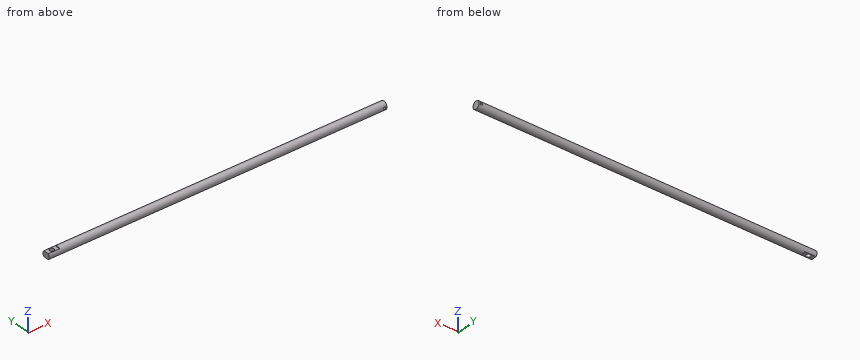
from build123d import *

# Parameters (mm, degrees)
SKETCH_1_R           = 7
EXTRUDE_1_DEPTH      = 600
SKETCH_3_OUTSIDE_W   = 136.066
SKETCH_3_OUTSIDE_H   = 136.066
SKETCH_3_OUTSIDE_W_2 = 10
SKETCH_3_OUTSIDE_H_2 = 20
CUT_EXTRUDE_1_DEPTH  = 20
SKETCH_4_R           = 4
CUT_EXTRUDE_3_DEPTH  = 20
SKETCH_5_R           = 2
CUT_EXTRUDE_4_DEPTH  = 15


with BuildPart() as part:
    # 草图1 → 凸台-拉伸1 (new body)
    with BuildSketch(Plane(origin=(0, 0, 0), x_dir=(0, 0, -1), z_dir=(1, 0, 0))):
        Circle(SKETCH_1_R)
    extrude(amount=EXTRUDE_1_DEPTH)

    # 草图3 outside → 切除-拉伸1 (cut)
    with BuildSketch(Plane.ZY):
        Rectangle(SKETCH_3_OUTSIDE_W, SKETCH_3_OUTSIDE_H)
        Rectangle(SKETCH_3_OUTSIDE_W_2, SKETCH_3_OUTSIDE_H_2, mode=Mode.SUBTRACT)
    extrude(amount=-CUT_EXTRUDE_1_DEPTH, mode=Mode.SUBTRACT)

    # 草图4 → 切除-拉伸3 (cut)
    with BuildSketch(Plane(origin=(0, 0, -5), x_dir=(-1, 0, 0), z_dir=(0, 0, -1))):
        with Locations((-10, 0)):
            Circle(SKETCH_4_R)
    extrude(amount=-CUT_EXTRUDE_3_DEPTH, mode=Mode.SUBTRACT)

    # 草图5 → 切除-拉伸4 (cut, through all)
    with BuildSketch(Plane(origin=(-583.138159927, 7, 1388.026133711), x_dir=(-1, 0, 0), z_dir=(0, 1, 0))):
        with Locations((-1179.138160513, -1388.026133214)):
            Circle(SKETCH_5_R)
    extrude(amount=-CUT_EXTRUDE_4_DEPTH, mode=Mode.SUBTRACT)


solid = part.part
CAD build for the part. Positions are in the model's coordinates, mm. Round coordinates to 2 decimals unless told otherwise and drop trailing zeros. Write each loop counter-clockwise with the first axis right and the second up, starting at its lowest first coordinate (ties: lowest second). Pieces come first, ordered by that corner, then holes.
(1) Probe line 1 along X through (y, z) = (-5, -0.5); line 2 along Y through (x, z) = (10, 0.75); line 3 along Z through (x, y) = (596, -0.5). List the from-to ranges inside material, lowest first.
(2) Drop flat-ended pins along their axis: P1, Ø6, axis at x = 100, y = 3, coming from the +Z side; P2, Ø3, axis at x = 12.5, y = 1, coming from the +Z side; P3, Ø8, axis at x = 6, y = -1.5, coming from the -Z side; P4, Ø0.6, axis at y = -2, z = -6.5, coming from the -X side. Give the stop position or say it passes through.
(3) Slice it at A-A, the plane x = 295. Write the cut outline in (y, z).
From the geometry:
1. line 1: x = 0 to 594.06, 597.94 to 600
1. line 2: y = -6.96 to -4, 4 to 6.96
1. line 3: z = -6.98 to -2, 2 to 6.98
2. P1: stops at z = 7
2. P2: stops at z = 5
2. P3: stops at z = -5
2. P4: stops at x = 20
3. outline: circle Ø14 at (0, 0)
